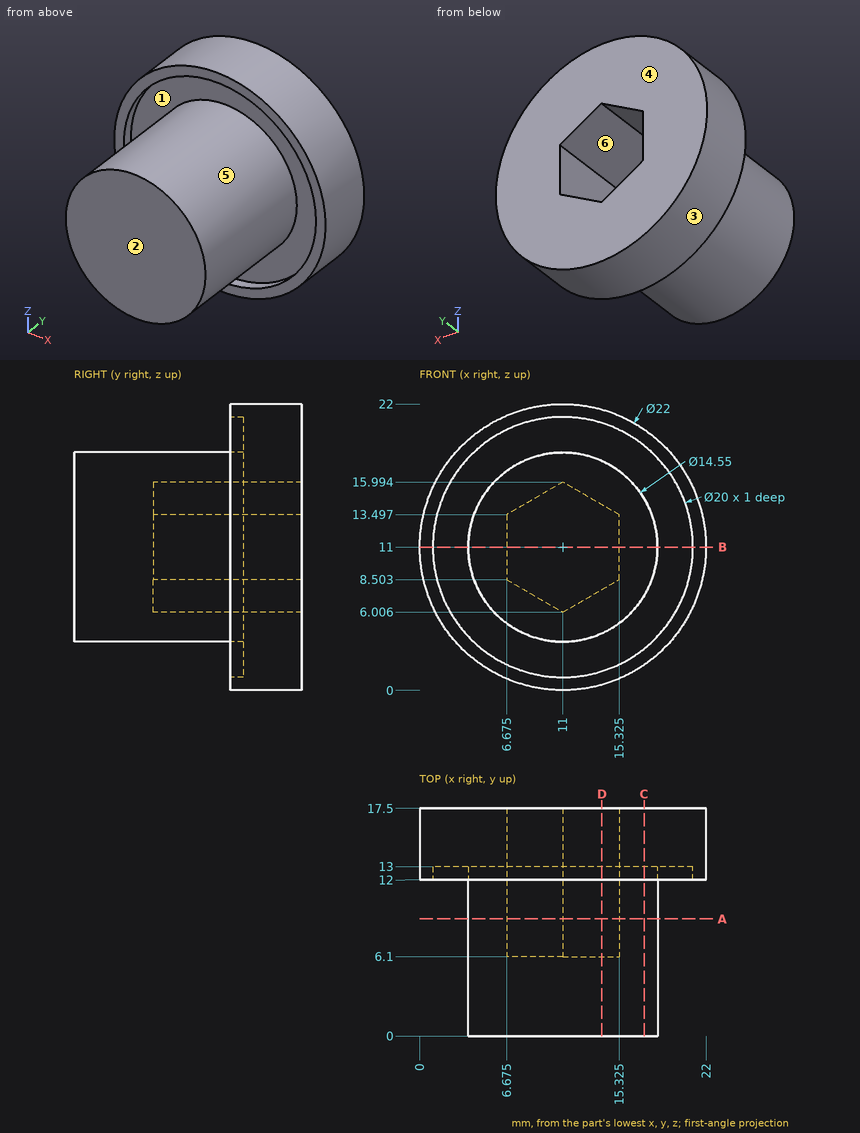
Job drawing, mm, ordinate dimensions from the low corner. One solid piece. A direction names the side the tool comes from. Give positions to 0.01 mm unless a question says otherwise; leave off trailing zeros. Loops run counter-clockwise (first coordinate to the right, second up) from the corner with the lowest first, then second, coordinate; pieces in that order, holes last. Notation, with made-up numbers: (15.5, -8) - (70.5, -8) arc R13 cw to (70.5, 13) - close; hole circle Ø4 at (12.5, 89.25). An arc over 180 degrees is marked (long way). Use one line per item in the form item = value.
(1) Cut at D-D (x = 14). Give the cut face in (y, z).
Determined:
outline = (0, 4.37) - (13, 4.37) - (13, 1.46) - (12, 1.46) - (12, 0.42) - (17.5, 0.42) - (17.5, 7.74) - (6.1, 7.74) - (6.1, 14.26) - (17.5, 14.26) - (17.5, 21.58) - (12, 21.58) - (12, 20.54) - (13, 20.54) - (13, 17.63) - (0, 17.63) - close
(2) 3-axis set-ups, long thin cutter, end or side, ignore diameter. For the marked faces 4, 5 and 6: which of +Z, -Z, +X, -X, +Y, -Y reach the whole face in a straight line?
Determined:
face_4 = +Z, -Z, +X, -X, +Y
face_5 = -Y
face_6 = +Y
(3) Drill centre lines: L1, parallel to Z at x = 8.5, y = 7.75; L2, parallel to Y at x = 13, z = 2.75; L3, parallel to Z at x = 11.5, y = 11.75 (1 decimal). Where is each one in solid material? Low to high.
Determined:
L1 = 4.17 to 7.45, 14.55 to 17.83
L2 = 13 to 17.5
L3 = 3.7 to 6.3, 15.7 to 18.3
(4) Cut at B-B (z = 11). Give the cut face in (x, y) (3 decimals), then the cut area to 3 significant figures.
Determined:
outline = (0, 12) - (1, 12) - (1, 13) - (3.725, 13) - (3.725, 0) - (18.275, 0) - (18.275, 13) - (21, 13) - (21, 12) - (22, 12) - (22, 17.5) - (15.325, 17.5) - (15.325, 6.1) - (6.675, 6.1) - (6.675, 17.5) - (0, 17.5) - close
area = 192 mm^2
(5) Drop flat-ended pins along their axis: P1, Ø2, axis at x = 9, z = 5, coming from the -Y side; P2, Ø3, axis at x = 5.5, y = 15, coming from the -Z side; P3, Ø1.5, axis at x = 4.5, y = 4, coming from the -Z side; P4, Ø4, axis at x = 8.5, y = 5, coming from the +Z side. Give the stop position or say it passes through.
Determined:
P1 = 0
P2 = 0.75
P3 = 6.54
P4 = 18.26
(6) Cut at C-C (x = 17.25). Give the cut face in (y, z), then the cut area to 3 significant figures.
Determined:
outline = (0, 7.28) - (13, 7.28) - (13, 3.19) - (12, 3.19) - (12, 1.95) - (17.5, 1.95) - (17.5, 20.05) - (12, 20.05) - (12, 18.81) - (13, 18.81) - (13, 14.72) - (0, 14.72) - close
area = 181 mm^2
(7) Cut at A-A (y = 9). Give the cut face in (x, z) (3 decimals), then the cut area to 3 significant figures.
Determined:
outline = circle Ø14.55 at (11, 11); hole (6.675, 8.503) - (11, 6.006) - (15.325, 8.503) - (15.325, 13.497) - (11, 15.994) - (6.675, 13.497) - close
area = 101 mm^2
(8) Pull direction Z, two halves, no side cores. Call the marked faces 1, 2 and 3: pulls with the +Z half, pulls with the -Z half, needs draft (parallel to the pull), parting line crosses it, or undercut.
Determined:
face_1 = undercut
face_2 = needs draft
face_3 = parting line crosses it
